Work out the finished part from the listing and answer in its coordinate system (mm). A direction names the side the tool comes from. Round coordinates to 2 decimals unless told otherwise and drop trailing zeros. Write each loop counter-clockwise with the first axis right and the second up, starting at its lowest first coordinate (ties: lowest second). Pieces come first, ordered by that corner, then holes. Notation, with made-up numbers: (44.25, 72) -> (81.25, 72) arc R19 cw to (81.25, 105) -> close; hole circle Ø4 at (89, 67). An arc over 180 degrees is marked (long way). One line per question, with ' | ' between items. Start each with the question number.
```python
from build123d import *

# Parameters (mm, degrees)
SKETCH1_W               = 172.72
SKETCH1_H               = 73.66
SKETCH1_R               = 1.63195
BOSS_EXTRUDE1_DEPTH     = 6.35
SKETCH2_W               = 88.9
SKETCH2_H               = 44.45
CUT_EXTRUDE1_DEPTH      = 6.35
FILLET1_R               = 2.54
BOSS_EXTRUDE2_DEPTH     = 3.81
CHAMFER1_SIZE           = 2.54
CHAMFER2_SIZE           = 2.54
CUT_EXTRUDE3_DEPTH      = 189.045791232
CUT_EXTRUDE3_DEPTH_BACK = 2.54
CUT_EXTRUDE4_DEPTH      = 189.045791232
CUT_EXTRUDE4_DEPTH_BACK = 2.54
SKETCH8_R               = 5.08
BOSS_EXTRUDE3_DEPTH     = 2.54
SKETCH9_R               = 1.9685
CUT_EXTRUDE5_DEPTH      = 6.35
SKETCH10_W              = 134.62
SKETCH10_H              = 2.54
SKETCH10_W_2            = 114.3
SKETCH10_W_3            = 2.54
SKETCH10_H_2            = 35.56
SKETCH10_H_3            = 52.197
SKETCH10_W_4            = 6.35
BOSS_EXTRUDE4_DEPTH     = 3.81
FILLET2_R               = 2.54


with BuildPart() as part:
    # Sketch1 → Boss-Extrude1 (new body)
    with BuildSketch(Plane(origin=(0, 0, 0), x_dir=(1, 0, 0), z_dir=(0, 1, 0))):
        with Locations((86.36, 36.83)):
            Rectangle(SKETCH1_W, SKETCH1_H)
        with Locations(Location((24.765, 66.675, 0), (0, 0, 270))):
            Circle(SKETCH1_R, mode=Mode.SUBTRACT)
        with Locations(Location((8.89, 8.89, 0), (0, 0, 270))):
            Circle(SKETCH1_R, mode=Mode.SUBTRACT)
        with Locations(Location((163.83, 66.675, 0), (0, 0, 270))):
            Circle(SKETCH1_R, mode=Mode.SUBTRACT)
        with Locations(Location((163.83, 8.89, 0), (0, 0, 270))):
            Circle(SKETCH1_R, mode=Mode.SUBTRACT)
    extrude(amount=BOSS_EXTRUDE1_DEPTH)

    # Sketch2 → Cut-Extrude1 (cut)
    with BuildSketch(Plane(origin=(0, 6.35, 0), x_dir=(1, 0, 0), z_dir=(0, 1, 0))):
        with Locations((57.15, 37.465)):
            Rectangle(SKETCH2_W, SKETCH2_H)
    extrude(amount=-CUT_EXTRUDE1_DEPTH, mode=Mode.SUBTRACT)

    # Fillet1
    fillet1_edges = [part.edges().sort_by_distance(p)[0] for p in [
        (172.72, 6.35, -36.83),
        (86.36, 6.35, -73.66),
        (0, 6.35, -36.83),
        (0, 3.175, -73.66),
        (172.72, 3.175, -73.66),
        (172.72, 3.175, 0),
        (0, 3.175, 0),
        (86.36, 6.35, 0),
    ]]
    fillet(fillet1_edges, radius=FILLET1_R)

    # Sketch3 → Boss-Extrude2 (add)
    with BuildSketch(Plane.XZ):
        Polygon((10.16, -12.7), (104.14, -12.7), (104.14, -17.78), (15.24, -17.78), (15.24, -26.67), (10.16, -26.67), align=None)
        Polygon((10.16, -62.23), (104.14, -62.23), (104.14, -57.15), (15.24, -57.15), (15.24, -48.26), (10.16, -48.26), align=None)
    extrude(amount=BOSS_EXTRUDE2_DEPTH)

    # Chamfer1
    chamfer1_edges = [part.edges().sort_by_distance(p)[0] for p in [
        (12.7, 0, -37.465),
    ]]
    chamfer(chamfer1_edges, length=CHAMFER1_SIZE)

    # Chamfer2
    chamfer2_edges = [part.edges().sort_by_distance(p)[0] for p in [
        (58.42, 0, -17.78),
        (15.24, 0, -22.225),
        (15.24, 0, -52.705),
        (58.42, 0, -57.15),
    ]]
    chamfer(chamfer2_edges, length=CHAMFER2_SIZE - 0.0001)  # a hair under: the kernel refuses the full size

    # Sketch6 → Cut-Extrude3 (cut, two sides: drawn at the far end of the back side and taken through both)
    with BuildSketch(Plane(origin=(0, 6.35, 0), x_dir=(1, 0, 0), z_dir=(0, 1, 0)).offset(-CUT_EXTRUDE3_DEPTH_BACK)):
        with BuildLine():
            ThreePointArc((114.299859558, 37.422767419), (112.462469481, 41.932674919), (107.971116407, 43.814964889))
            Line((107.971116407, 43.814964889), (107.928883593, 43.814964889))
            ThreePointArc((107.928883593, 43.814964889), (103.452412358, 41.947656066), (101.6, 37.465))
            Line((101.6, 37.465), (101.6, 21.589866304))
            ThreePointArc((101.6, 21.589866304), (103.329230599, 17.234296291), (107.575115004, 15.250942007))
            Line((107.575115004, 15.250942007), (108.348372102, 15.252374712))
            ThreePointArc((108.348372102, 15.252374712), (112.842425973, 17.541821331), (114.250015644, 22.385041059))
            Line((114.250015644, 22.385041059), (114.299859558, 37.422767419))
        make_face()
    extrude(amount=CUT_EXTRUDE3_DEPTH + CUT_EXTRUDE3_DEPTH_BACK, mode=Mode.SUBTRACT)

    # Sketch7 → Cut-Extrude4 (cut, two sides: drawn at the far end of the back side and taken through both)
    with BuildSketch(Plane(origin=(0, 6.35, 0), x_dir=(1, 0, 0), z_dir=(0, 1, 0)).offset(-CUT_EXTRUDE4_DEPTH_BACK)):
        with BuildLine():
            Line((101.6, 43.68515436), (101.6, 37.465))
            ThreePointArc((101.6, 37.465), (103.362031135, 41.855107253), (107.670249351, 43.808834769))
            Line((107.670249351, 43.808834769), (101.6, 43.68515436))
        make_face()
        with BuildLine():
            ThreePointArc((107.563787548, 15.251622072), (103.325340603, 17.238426833), (101.6, 21.589866304))
            Line((101.6, 21.589866304), (101.6, 15.24))
            Line((101.6, 15.24), (107.563787548, 15.251622072))
        make_face()
    extrude(amount=CUT_EXTRUDE4_DEPTH + CUT_EXTRUDE4_DEPTH_BACK, mode=Mode.SUBTRACT)

    # Sketch8 → Boss-Extrude3 (add)
    with BuildSketch(Plane.XZ):
        with Locations(Location((107.95, -37.465, 0), (0, 0, 90))):
            Circle(SKETCH8_R)
    extrude(amount=BOSS_EXTRUDE3_DEPTH)

    # Sketch9 → Cut-Extrude5 (cut)
    with BuildSketch(Plane.XZ.offset(2.54)):
        with Locations(Location((107.95, -37.465, 0), (0, 0, 270))):
            Circle(SKETCH9_R)
    extrude(amount=-CUT_EXTRUDE5_DEPTH, mode=Mode.SUBTRACT)

    # Sketch10 → Boss-Extrude4 (add)
    with BuildSketch(Plane.XZ):
        with Locations((86.36, -5.588)):
            Rectangle(SKETCH10_W, SKETCH10_H)
        with Locations((96.52, -69.977)):
            Rectangle(SKETCH10_W_2, SKETCH10_H)
        with Locations((167.132, -36.83)):
            Rectangle(SKETCH10_W_3, SKETCH10_H_2)
        with Locations((5.588, -45.1485)):
            Rectangle(SKETCH10_W_3, SKETCH10_H_3)
        with Locations((10.033, -69.977)):
            Rectangle(SKETCH10_W_4, SKETCH10_H)
    extrude(amount=BOSS_EXTRUDE4_DEPTH)

    # Fillet2
    fillet2_edges = [part.edges().sort_by_distance(p)[0] for p in [
        (4.318, -1.905, -71.247),
    ]]
    fillet(fillet2_edges, radius=FILLET2_R)


solid = part.part
```
(1) Given pin 1 Ø3 at (y, z) = (-2.5, -15.5) entering from +X; pin 2 Ø0.8 at (y, z) = (-2, -69.5) entering from +X; pin 3 Ø0.8 at (x, y) = (6, -2.5) entering from +Z, each flat-ended and moving along its own axis, determine where each tip first touches the part or whether it passes through.
(2) A cutting plane is placed at C-C, the plane x = 120.5. Determine the outline of the cut face in (y, z), then the cut area to 3 significant figures.
(3) Consider L1, parallel to X at y = 1.5, z = -8.89; L2, parallel to Z at x = 163.83, y = 3; L3, parallel to X at y = -0.5, z = -27. Determine where each line is inside the solid, lowest interval first.
(4) The mould has two halves that part along X. Classify faces 1 (the flat face through (165.862, -2, -37)), 2 (the flat face through (46, -3.81, -58)), 3 (the flat face through (0, 2, -36)): +X half, -X half, draft (parallel to the pull), parting line (faces both ways), or undercut.
(5) A cutting plane is placed at B-B, the plane z = -8.89. Determine the outline of the cut face in (x, y).
(6) For faces 4 (the flat face through (56, -2, -62.23)), 5 (the cylindrical face through (112.511, 5.062, -41.883)), 6 (the flat face through (85, -2, -4.318)), 7 (the flat face through (108, -2.54, -35)), determine the directions among +Z, -Z, +X, -X, +Y, -Y from which every point of the face is accessible in a straight line to the end or side of a thin tool.
Returned:
1) pin 1: x = 104.14 | pin 2: x = 153.67 | pin 3: z = -19.05
2) outline: (-3.81, -71.25) -> (0, -71.25) -> (0, -73.66) -> (3.81, -73.66) arc R2.54 ccw to (6.35, -71.12) -> (6.35, -2.54) arc R2.54 ccw to (3.81, 0) -> (0, 0) -> (0, -4.32) -> (-3.81, -4.32) -> (-3.81, -6.86) -> (0, -6.86) -> (0, -68.71) -> (-3.81, -68.71) -> close | area: 484 mm2
3) L1: 0 to 7.26, 10.52 to 162.2, 165.46 to 172.72 | L2: -73.66 to -68.31, -65.04 to -10.52, -7.26 to 0 | L3: 4.32 to 6.86, 165.86 to 168.4
4) face 1: undercut | face 2: draft | face 3: -X half
5) outline: (0, 0) -> (7.26, 0) -> (7.26, 6.35) -> (2.54, 6.35) arc R2.54 ccw to (0, 3.81) -> close; (10.52, 0) -> (162.2, 0) -> (162.2, 6.35) -> (10.52, 6.35) -> close; (165.46, 0) -> (172.72, 0) -> (172.72, 3.81) arc R2.54 ccw to (170.18, 6.35) -> (165.46, 6.35) -> close
6) face 4: +X, -Y | face 5: +Y | face 6: +Z, +X, -X, -Y | face 7: -Y
